Read the model definition and answer for the solid it produces. Units are mm, in the model's axes. Face numbers are marked on the shaded views. Give positions to 0.01 mm unless a question says otherwise; leave off trailing zeros. Order: outer loops, then holes, each group sorted by start corner. A loop starts at its lowest first (then second) coordinate and runs counter-clockwise, first axis right, second up.
Item 1: A cutting plane is placed at B-B (x = 5). Write down the section's boundary in (y, z), plus the area to 3 significant figures.
Item 2: A cutting plane is placed at A-A (z = -4.25). Write down the section's boundary in (x, y).
Item 3: Given pin 1 Ø3 at (x, y) = (5.5, 4) entering from +Z, flat-ended and moving along its own axis, determine where the tip first touches the part or whether it passes through.
Item 4: The mould has two halves that part along Y. Classify the marked faces 1, 2 and 3: +Y half, -Y half, draft (parallel to the pull), parting line (faces both ways), or undercut.
Item 5: Find the intervals of material crossed by line 1 along X through (y, z) = (5, -2.3); line 2 along Z through (x, y) = (4.75, 7.5), in increasing order.
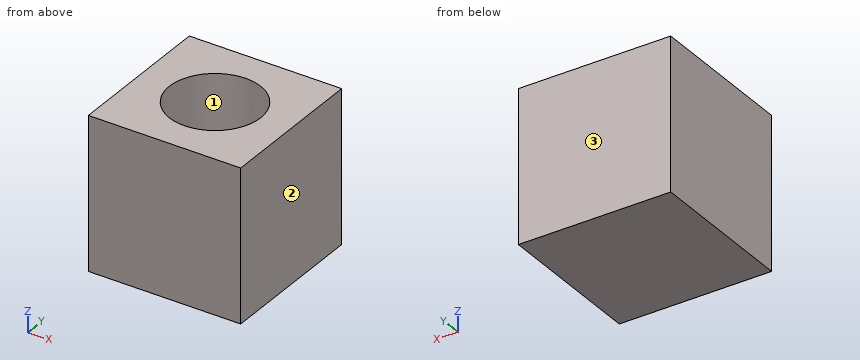
from build123d import *

# Parameters (mm, degrees)
CYLINDER_R     = 3
CYLINDER_DEPTH = 10
BOX_W          = 10
BOX_H          = 10
BOX_DEPTH      = 10


with BuildPart() as cylinder:
    # Cylinder → Cylinder (new body)
    with BuildSketch(Plane(origin=(5, 5, 5), x_dir=(1, 0, 0), z_dir=(0, 0, 1))):
        Circle(CYLINDER_R)
    extrude(amount=CYLINDER_DEPTH)


with BuildPart() as model_cut:
    # Box → Box (new body)
    with BuildSketch(Plane.XY):
        with Locations((5, 5)):
            Rectangle(BOX_W, BOX_H)
    extrude(amount=BOX_DEPTH)

    # Cut: cut Cylinder
    add(cylinder.part, mode=Mode.SUBTRACT)


with BuildPart() as model_cut_1:
    # Clone placement: moved
    add(model_cut.part.moved(Location((0, 0, -10))))


solid = model_cut_1.part
Response values:
1. outline: (0, -10) - (10, -10) - (10, 0) - (8, 0) - (8, -5) - (2, -5) - (2, 0) - (0, 0) - close
1. area: 70.0 mm2
2. outline: (0, 0) - (10, 0) - (10, 10) - (0, 10) - close; hole circle Ø6 at (5, 5)
3. pin 1: stops at z = -5
4. face 1: undercut
4. face 2: draft
4. face 3: +Y half
5. line 1: x = 0 to 2, 8 to 10
5. line 2: z = -10 to -5
